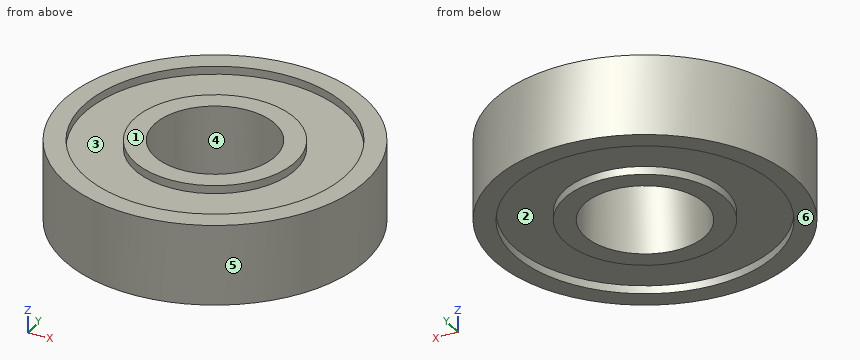
Autodesk Inventor part; units mm, degrees
ref_plane "YZ Plane" through (0, 0, 0) normal (1, 0, 0) x (0, 1, 0)
ref_plane "XZ Plane" through (0, 0, 0) normal (0, 1, 0) x (-1, 0, 0)
ref_plane "XY Plane" through (0, 0, 0) normal (0, 0, 1) x (1, 0, 0)
sketch "Boceto1" plane through (0, 0, 0) normal (1, 0, 0) x (0, 1, 0)
  line L0 (0, 30.1209) -> (0, -30.1209) construction
  line L1 (15, 4) -> (15, -4)
  line L2 (15, -4) -> (13, -4)
  line L3 (13, -4) -> (13, -3.2)
  line L4 (13, -3.2) -> (8, -3.2)
  line L5 (8, -3.2) -> (8, -4)
  line L6 (8, -4) -> (6, -4)
  line L7 (6, -4) -> (6, 4)
  line L8 (6, 4) -> (8, 4)
  line L9 (8, 4) -> (8, 3.2)
  line L10 (8, 3.2) -> (13, 3.2)
  line L11 (13, 3.2) -> (13, 4)
  line L12 (15, 4) -> (13, 4)
  circle A0 centre (10.5, 0) radius 2.2
  point P0 (0, 0)
  point P1 (0, 0)
  point P2 (6, 0)
  point P3 (10.5, -3.2)
  dimension "d0" = 1
  dimension "d1" = 0.3
  dimension "d2" = 30
  dimension "d3" = 8
  dimension "d4" = 0.8
  dimension "d5" = 2
  dimension "d6" = 12
revolve "Revolución1" add sketch "Boceto1" angle 360 about axis through (0, 0, 30.1209) along (0, 0, -1)
properties part number "rodamiento"
Build history of the part. All positions in model axes, mm. Face numbers are marked on the shaded views. A direction names the side the tool comes from. Coordinates: 2 decimals unless noted, no trailing zeros. Order: outer loops, then holes, each group sorted by start corner. A loop starts at its lowest first (then second) coordinate and runs counter-clockwise, first axis right, second up.
Item 1: Tool access for the marked faces 1 and 2: list every direction of +Z, -Z, +X, -X, +Y, -Y with a clear straight run to the whole face (end or side of a thin tool).
Filled in:
face 1: +Z, +X, -X, +Y, -Y
face 2: -Z
Item 2: Drop flat-ended pins along their axis: pin 1 Ø2 at (x, y) = (9, 3) entering from -Z; pin 2 Ø10 at (x, y) = (-11, 5) entering from -Z; pin 3 Ø2 at (y, z) = (5, -2.5) entering from +X; pin 4 Ø2 at (x, z) = (3, 2.5) entering from -Y. Give the stop position or say it passes through.
Filled in:
pin 1: stops at z = -3.2
pin 2: stops at z = -4
pin 3: stops at x = 14.46
pin 4: stops at y = -14.87
Item 3: Drill centre lines: L1, parallel to X at y = 0, z = -3.5; L2, parallel to Y at x = 5.25, z = 1.5; L3, parallel to Z at x = -10, y = -3.5. Where is each one in solid material? Low to high.
Filled in:
L1: x = -15 to -13, -8 to -6, 6 to 8, 13 to 15
L2: y = -14.05 to -10.91, -7.18 to -2.9, 2.9 to 7.18, 10.91 to 14.05
L3: z = -3.2 to -2.2, 2.2 to 3.2
Item 4: Mould opens along Y. For the marked faces 3, 4, 5 and 6 say: released by +Y, released by -Y, zero draft, split by the parting line, or undercut.
Filled in:
face 3: undercut
face 4: undercut
face 5: split by the parting line
face 6: zero draft
Item 5: Saw through at A-A on y = 0. List the corners of the cut face in (x, z), then the cut area to 3 significant figures.
Filled in:
outline: (-15, -4) - (-13, -4) - (-13, -3.2) - (-8, -3.2) - (-8, -4) - (-6, -4) - (-6, 4) - (-8, 4) - (-8, 3.2) - (-13, 3.2) - (-13, 4) - (-15, 4) - close; (6, -4) - (8, -4) - (8, -3.2) - (13, -3.2) - (13, -4) - (15, -4) - (15, 4) - (13, 4) - (13, 3.2) - (8, 3.2) - (8, 4) - (6, 4) - close; hole circle Ø4.4 at (-10.5, 0); hole circle Ø4.4 at (10.5, 0)
area: 97.6 mm2
